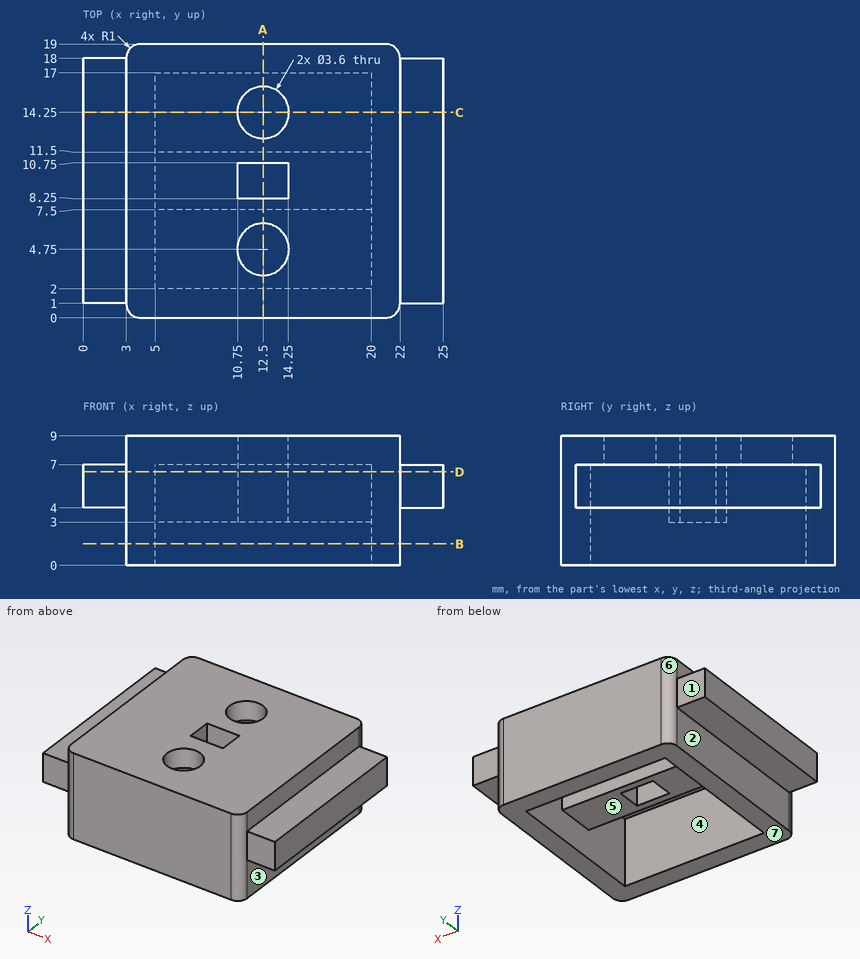
Here's the drawing with two shaded views (mm, measured from the low corner). I have some questions. A direction names the side the tool comes from. Coordinates: 2 decimals unless noted, no trailing zeros. Order: outer loops, then holes, each group sorted by start corner. A loop starts at its lowest first (then second) coordinate and runs counter-clockwise, first axis right, second up.
Item 1: If we section it at D-D on z = 6.5: List the corners of the cut face in (x, y) for me, plus the area to 3 significant figures.
Result sheet:
outline: (0, 1) - (3, 1) arc R1 ccw to (4, 0) - (21, 0) arc R1 ccw to (22, 1) - (25, 1) - (25, 18) - (22, 18) arc R1 ccw to (21, 19) - (4, 19) arc R1 ccw to (3, 18) - (0, 18) - close; hole (5, 2) - (20, 2) - (20, 7.5) - (5, 7.5) - close; hole (5, 11.5) - (20, 11.5) - (20, 17) - (5, 17) - close; hole (10.75, 8.25) - (14.25, 8.25) - (14.25, 10.75) - (10.75, 10.75) - close
area: 288 mm2
Item 2: For P1, Ø1.5, axis at x = 9.5, z = 8, coming from the -Y side; P2, Ø3, axis at y = 5.5, z = 2, coming from the -X side; P3, Ø1.5, axis at x = 24, y = 7, coming from the -Z side; P4, Ø4.5, axis at x = 13, y = 10.5, coming from the -Z side, each with a flat end and sliding along its axis, tell me the tip position at first contact or that it passes through.
Result sheet:
P1: stops at y = 0
P2: stops at x = 3
P3: stops at z = 4
P4: stops at z = 3
Item 3: If we mould it in two halves opening along X, with no side actions, what happens to the marked faces 5, 6 and 7? For each: +X half, -X half, draft (parallel to the pull), parting line (faces both ways), or undercut.
Result sheet:
face 5: undercut
face 6: -X half
face 7: draft
Item 4: For the marked faces 1, 2, 3 and 4, which set-ups out of +Z, -Z, +X, -X, +Y, -Y let a thin tool reach every point of the face, with its end or its side?
Result sheet:
face 1: +Z, -Z, -X, +Y
face 2: -Z, -X, +Y, -Y
face 3: -Z, +X, +Y, -Y
face 4: -Z
Item 5: If we section it at B-B on z = 1.5: List the corners of the cut face in (x, y) for me, plus the area to 3 significant figures.
Result sheet:
outline: (3, 1) arc R1 ccw to (4, 0) - (21, 0) arc R1 ccw to (22, 1) - (22, 18) arc R1 ccw to (21, 19) - (4, 19) arc R1 ccw to (3, 18) - close; hole (5, 2) - (20, 2) - (20, 17) - (5, 17) - close
area: 135 mm2
Item 6: If we section it at A-A on x = 12.5: List the corners of the cut face in (y, z) for me, plus the area to 3 significant figures.
Result sheet:
outline: (0, 0) - (2, 0) - (2, 7) - (2.95, 7) - (2.95, 9) - (0, 9) - close; (6.55, 7) - (7.5, 7) - (7.5, 3) - (8.25, 3) - (8.25, 9) - (6.55, 9) - close; (10.75, 3) - (11.5, 3) - (11.5, 7) - (12.45, 7) - (12.45, 9) - (10.75, 9) - close; (16.05, 7) - (17, 7) - (17, 0) - (19, 0) - (19, 9) - (16.05, 9) - close
area: 52.6 mm2
Item 7: I need wall thicknesses on line 1 (Y direction, x = 12.5, z = 7.5); line 2 (X direction, y = 14.25, z = 8.1); line 3 (Y direction, x = 11, z = 5.75). Which ranges of each line are inside material? Lowest first, please.
Result sheet:
line 1: y = 0 to 2.95, 6.55 to 8.25, 10.75 to 12.45, 16.05 to 19
line 2: x = 3 to 10.7, 14.3 to 22
line 3: y = 0 to 2, 7.5 to 8.25, 10.75 to 11.5, 17 to 19
Item 8: If we section it at C-C on y = 14.25: List the corners of the cut face in (x, z) for me, plus the area to 3 significant figures.
Result sheet:
outline: (0, 4) - (3, 4) - (3, 0) - (5, 0) - (5, 7) - (10.7, 7) - (10.7, 9) - (3, 9) - (3, 7) - (0, 7) - close; (14.3, 7) - (20, 7) - (20, 0) - (22, 0) - (22, 4) - (25, 4) - (25, 7) - (22, 7) - (22, 9) - (14.3, 9) - close
area: 76.8 mm2
